The drawing under review shows one solid part. Ordinate dimensions are in mm from its lowest x, y, z. Coordinates: 2 decimals unless noted, no trailing zeros. Order: outer loops, then holes, each group sorted by start corner. A loop starts at its lowest first (then second) coordinate and runs counter-clockwise, first axis right, second up. Notation, with made-up numbers: (54, 46.25) -> (61, 46.25) arc R31 ccw to (61, 81.25) -> close; hole circle Ø7 at (-1, 46.5). An arc over 180 degrees is marked (long way). Write item = value, one per line.
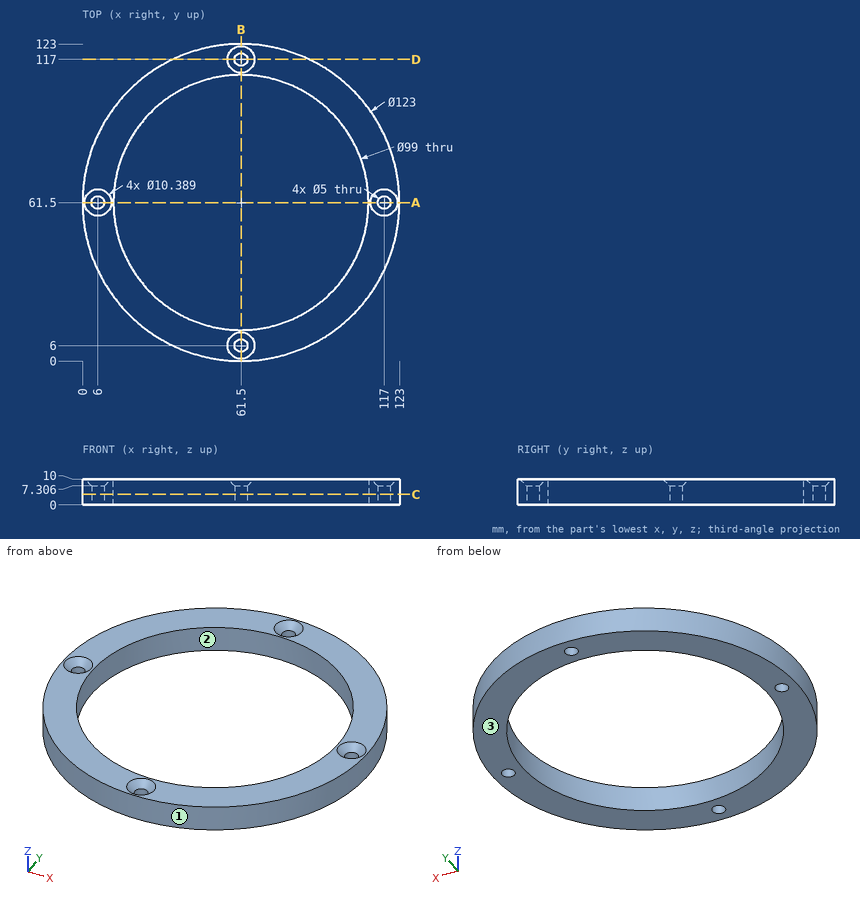
(1) We need section C-C (z = 4). Write out the cut boundary in (x, y).
Report:
outline = circle Ø123 at (61.5, 61.5); hole circle Ø5 at (6, 61.5); hole circle Ø99 at (61.5, 61.5); hole circle Ø5 at (61.5, 6); hole circle Ø5 at (61.5, 117); hole circle Ø5 at (117, 61.5)
(2) We need section A-A (y = 61.5). Write out the cut boundary in (x, z) (1 decimal).
Report:
outline = (0, 0) -> (3.5, 0) -> (3.5, 7.3) -> (0.8, 10) -> (0, 10) -> close; (8.5, 0) -> (12, 0) -> (12, 10) -> (11.2, 10) -> (8.5, 7.3) -> close; (111, 0) -> (114.5, 0) -> (114.5, 7.3) -> (111.8, 10) -> (111, 10) -> close; (119.5, 0) -> (123, 0) -> (123, 10) -> (122.2, 10) -> (119.5, 7.3) -> close
(3) Insertion check: pin 1 (4 mm diameter, centred on y = 25, z = 2, fed in from -X); pin 2 (1.5 mm diameter, centred on x = 60, z = 4.5, fed in from -Y) (1 decimal); pin 3 (6 mm diameter, centred on y = 33.5, z = 3.5, fed in from +X). Each pin has a flat end and moves straight along its axis. Give the tip position at first contact, or say it passes through.
Report:
pin_1 = 10.59
pin_2 = 0
pin_3 = 117.69
(4) For L1, parallel to Y at x = 61.5, z = 3.25; L2, parallel to Y at x = 116, z = 3 (1 decimal); L3, parallel to Y at x = 50.5, z = 3.25, list the stretches that pass through material, from the lowest coordinate up.
Report:
L1 = 0 to 3.5, 8.5 to 12, 111 to 114.5, 119.5 to 123
L2 = 33 to 59.2, 63.8 to 90
L3 = 0.99 to 13.24, 109.76 to 122.01
(5) We need section D-D (y = 117). Write out the cut boundary in (x, z) (1 decimal), and give its area (3 significant figures).
Report:
outline = (35, 0) -> (59, 0) -> (59, 7.3) -> (56.3, 10) -> (35, 10) -> close; (64, 0) -> (88, 0) -> (88, 10) -> (66.7, 10) -> (64, 7.3) -> close
area = 473 mm²
(6) The part is to be moulded in two halves that separate along Y. For the marked faces 1, 2 and 3, say which applies: released by +Y, released by -Y, zero draft, split by the parting line, or undercut.
Report:
face_1 = split by the parting line
face_2 = undercut
face_3 = zero draft
